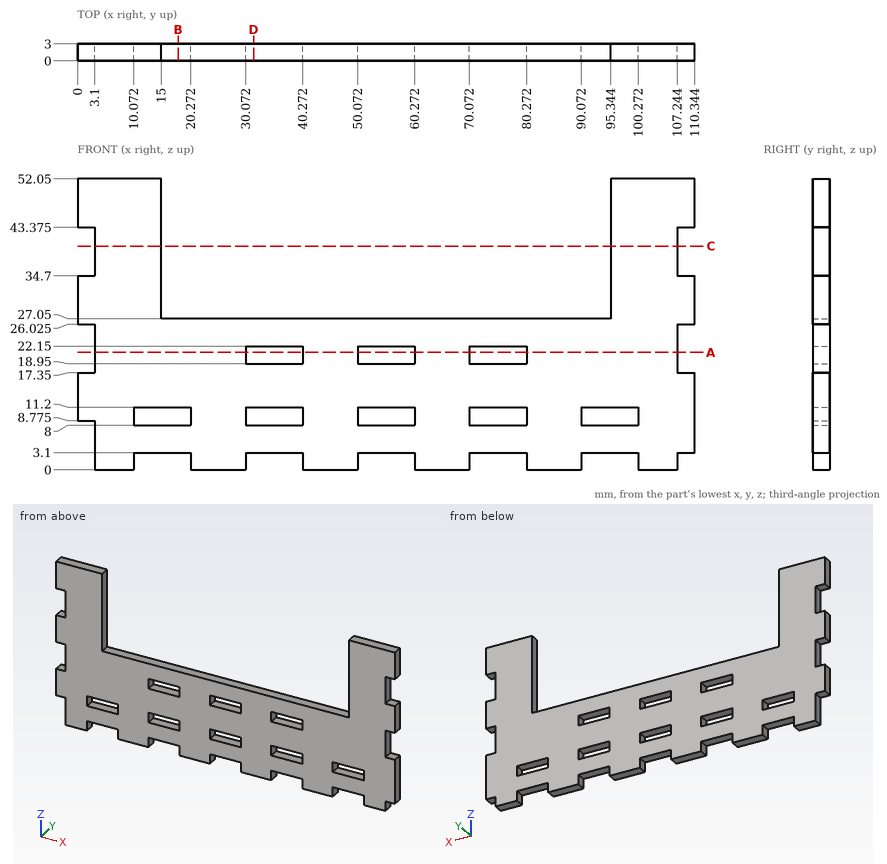
Part print with two shaded views. Sizes in mm from the minimum x, y, z corner. Give positions to 0.01 mm unless a question says otherwise; leave off trailing zeros. Order: outer loops, then holes, each group sorted by start corner. A loop starts at its lowest first (then second) coordinate and runs counter-clockwise, first axis right, second up.
1) Saw through at C-C, the plane z = 40. Write the cut outline in (x, y) (1 decimal).
2) Saw through at D-D, the plane x = 31.5. Write the cut outline in (y, z).
3) Wall check: probe 1 along X at (y, z) = (1.15, 2) (1 decimal); probe 2 along Z at (x, y) = (77.5, 0.6); probe 3 along X at (y, z) = (1.05, 19.5) (1 decimal). Give the ranges that are in metal, low to high.
4) Saw through at B-B, the plane x = 18. Write the cut outline in (y, z).
5) Pin check, flat tips, straight feed: pin 1 (0.9 mm diameter, centred on x = 36.5, y = 1, fed in from -Z); pin 2 (0.9 mm diameter, centred on y = 1, z = 1.5, fed in from -X); pin 3 (1.5 mm diameter, centred on x = 56.5, y = 1.5, fed in from +Z). Stop position of each tip, or through.
6) Saw through at A-A, the plane z = 21. Write the cut outline in (x, y) (1 decimal).
Computed:
1. outline: (3.1, 0) - (15, 0) - (15, 3) - (3.1, 3) - close; (95.3, 0) - (107.2, 0) - (107.2, 3) - (95.3, 3) - close
2. outline: (0, 3.1) - (3, 3.1) - (3, 8) - (0, 8) - close; (0, 11.2) - (3, 11.2) - (3, 18.95) - (0, 18.95) - close; (0, 22.15) - (3, 22.15) - (3, 27.05) - (0, 27.05) - close
3. probe 1: x = 3.1 to 10.1, 20.3 to 30.1, 40.3 to 50.1, 60.3 to 70.1, 80.3 to 90.1, 100.3 to 107.2
3. probe 2: z = 3.1 to 8, 11.2 to 18.95, 22.15 to 27.05
3. probe 3: x = 3.1 to 30.1, 40.3 to 50.1, 60.3 to 70.1, 80.3 to 107.2
4. outline: (0, 3.1) - (3, 3.1) - (3, 8) - (0, 8) - close; (0, 11.2) - (3, 11.2) - (3, 27.05) - (0, 27.05) - close
5. pin 1: stops at z = 3.1
5. pin 2: stops at x = 3.1
5. pin 3: stops at z = 27.05
6. outline: (3.1, 0) - (30.1, 0) - (30.1, 3) - (3.1, 3) - close; (40.3, 0) - (50.1, 0) - (50.1, 3) - (40.3, 3) - close; (60.3, 0) - (70.1, 0) - (70.1, 3) - (60.3, 3) - close; (80.3, 0) - (107.2, 0) - (107.2, 3) - (80.3, 3) - close
